from build123d import *

# Parameters (mm, degrees)
SKETCH1_W               = 15.2
SKETCH1_H               = 28
BOSS_EXTRUDE1_DEPTH     = 5.5
CUT_EXTRUDE1_DEPTH      = 14
CUT_EXTRUDE1_DEPTH_BACK = 12
SKETCH2_W               = 13.2
SKETCH2_H               = 5.5


with BuildPart() as part:
    # Sketch1 → Boss-Extrude1 (new body)
    with BuildSketch(Plane(origin=(0, 0, 0), x_dir=(1, 0, 0), z_dir=(0, 1, 0))):
        Rectangle(SKETCH1_W, SKETCH1_H)
    extrude(amount=BOSS_EXTRUDE1_DEPTH)

    # Sketch2 → Cut-Extrude1 (cut, two sides: drawn at the far end of the back side and taken through both)
    with BuildSketch(Plane.XY.offset(-CUT_EXTRUDE1_DEPTH_BACK)):
        with Locations((0, 4.75)):
            Rectangle(SKETCH2_W, SKETCH2_H)
    extrude(amount=CUT_EXTRUDE1_DEPTH + CUT_EXTRUDE1_DEPTH_BACK, mode=Mode.SUBTRACT)


solid = part.part
Work out the finished part from the listing and answer in its coordinate system (mm). A direction names the side the tool comes from. Give positions to 0.01 mm unless a question says otherwise; leave off trailing zeros. Write each loop counter-clockwise with the first axis right and the second up, starting at its lowest first coordinate (ties: lowest second). Pieces come first, ordered by that corner, then holes.
Q1. A tool of negligible diameter and unlimited length cuts with its end or side. For faces 1 (the face through (-7.6, 3, 0)), 2 (the face through (0, 2, 1)), from which of +Z, -Z, +X, -X, +Y, -Y can it reach the whole face along a straight path? Write none if from no direction.
Answer:
face 1: +Z, -Z, -X, +Y, -Y
face 2: +Z, +Y
Q2. For a pull along X with two mould halves and no side action, classify faces 3 (the face through (7.6, 3, 0)), 4 (the face through (0, 3, -14)), 5 (the face through (6.6, 4, 1)) as released by +X, released by -X, zero draft, split by the parting line, or undercut.
Answer:
face 3: released by +X
face 4: zero draft
face 5: undercut
Q3. The part is cut by section B-B on z = -10.5. Give the vertices of the cut face in (x, y), and give its area (3 significant figures).
Answer:
outline: (-7.6, 0) - (7.6, 0) - (7.6, 5.5) - (6.6, 5.5) - (6.6, 2) - (-6.6, 2) - (-6.6, 5.5) - (-7.6, 5.5) - close
area: 37.4 mm2
Q4. The part is cut by section A-A on y = 4.85. Give the vertices of the cut face in (x, z), and give its area (3 significant figures).
Answer:
outline: (-7.6, -14) - (7.6, -14) - (7.6, 14) - (6.6, 14) - (6.6, -12) - (-6.6, -12) - (-6.6, 14) - (-7.6, 14) - close
area: 82.4 mm2
Q5. Given pin 1 (4 mm diameter, centred on x = -2.5, z = 4, fed in from +Y), flat-ended and moving along its own axis, determine where the tip first touches the part or whether it passes through.
Answer:
pin 1: stops at y = 2
Q6. The part is cut by section C-C on x = -2.5. Give the vertices of the cut face in (y, z), and give its area (3 significant figures).
Answer:
outline: (0, -14) - (5.5, -14) - (5.5, -12) - (2, -12) - (2, 14) - (0, 14) - close
area: 63.0 mm2
Q7. Straight lines are drawn through the part: L1, parallel to X at y = 2.45, z = -3.5; L2, parallel to Z at x = 3.75, y = 4.25; L3, parallel to Y at x = -3.75, z = 7. For each, find the intervals that lie inside material, in ascending order.
Answer:
L1: x = -7.6 to -6.6, 6.6 to 7.6
L2: z = -14 to -12
L3: y = 0 to 2
